Check sheet for the modelled part. Datum: model origin and axes. Units: mm. A direction names the side the tool comes from. Give positions to 0.01 mm unless a question says otherwise; leave off trailing zeros. Order: outer loops, then holes, each group sorted by start corner. A loop starts at its lowest first (then second) coordinate and runs counter-clockwise, first axis right, second up. Notation, with made-up numbers: (-32.5, 19.5) -> (0.5, 19.5) arc R10 ccw to (0.5, 34.5) -> close; hole circle Ø10 at (62, 13.25). An arc over 180 degrees is marked (long way). One line per question, with ' | ' between items.
```python
from build123d import *

# Parameters (mm, degrees)
EXTRUDE_1_DEPTH              = 7
CUT_EXTRUDE_1_DEPTH          = 4
HOLE_WIZARD_M3_1_D           = 3.4
HOLE_WIZARD_M3_1_DEPTH       = 7.5
HOLE_WIZARD_M3_1_CSINK_D     = 6.72
HOLE_WIZARD_M3_1_CSINK_ANGLE = 90
HOLE_WIZARD_M3_1_TIP         = 1.021463052
HOLE_WIZARD_1_D              = 4.15
CUT_EXTRUDE_2_DEPTH          = 4
CHAMFER_1_SIZE               = 0.5


with BuildPart() as part:
    # 草图1 → 凸台-拉伸1 (new body)
    with BuildSketch(Plane(origin=(0, 0, 0), x_dir=(1, 0, 0), z_dir=(0, 1, 0))):
        with BuildLine():
            Line((0, 5), (9, 5))
            ThreePointArc((9, 5), (14, 0), (9, -5))
            Line((9, -5), (0, -5))
            ThreePointArc((0, -5), (-5, 0), (0, 5))
        make_face()
    extrude(amount=EXTRUDE_1_DEPTH)

    # 草图2 → 切除-拉伸1 (cut)
    with BuildSketch(Plane(origin=(0, 7, 0), x_dir=(1, 0, 0), z_dir=(0, 1, 0))):
        with BuildLine():
            ThreePointArc((-1.5, 2), (-2.5, 0), (-1.5, -2))
            Line((-1.5, -2), (1.5, -2))
            ThreePointArc((1.5, -2), (2.236067977, -1.118033989), (2.5, 0))
            ThreePointArc((2.5, 0), (2.236067977, 1.118033989), (1.5, 2))
            Line((1.5, 2), (-1.5, 2))
        make_face()
    extrude(amount=-CUT_EXTRUDE_1_DEPTH, mode=Mode.SUBTRACT)

    # M3 六角凹锥坑螺钉的锥形沉头孔1
    with Locations(Plane(origin=(0, 0, 0), x_dir=(-1, 0, 0), z_dir=(0, -1, 0))):
        with Locations((0, 0)):
            CounterSinkHole(HOLE_WIZARD_M3_1_D / 2, HOLE_WIZARD_M3_1_CSINK_D / 2, depth=HOLE_WIZARD_M3_1_DEPTH, counter_sink_angle=HOLE_WIZARD_M3_1_CSINK_ANGLE)
            with Locations((0, 0, -(HOLE_WIZARD_M3_1_DEPTH + HOLE_WIZARD_M3_1_TIP / 2))):  # 118° drill point
                Cone(0, HOLE_WIZARD_M3_1_D / 2, HOLE_WIZARD_M3_1_TIP, mode=Mode.SUBTRACT)

    # 孔1 (through all)
    with Locations(Plane(origin=(0, 0, 0), x_dir=(-1, 0, 0), z_dir=(0, -1, 0))):
        with Locations((-9, 0)):
            Hole(HOLE_WIZARD_1_D / 2)

    # 草图7 → 切除-拉伸2 (cut)
    with BuildSketch(Plane(origin=(0, 7, 0), x_dir=(1, 0, 0), z_dir=(0, 1, 0))):
        Polygon((12.348631561, 0), (10.674315781, 2.9), (7.325684219, 2.9), (5.651368439, 0), (7.325684219, -2.9), (10.674315781, -2.9), align=None)
    extrude(amount=-CUT_EXTRUDE_2_DEPTH, mode=Mode.SUBTRACT)

    # 倒角1
    chamfer_1_edges = [part.edges().sort_by_distance(p)[0] for p in [
        (14, 7, 0),
        (4.5, 7, -5),
        (-5, 7, 0),
        (4.5, 0, -5),
        (14, 0, 0),
        (4.5, 0, 5),
        (-5, 0, 0),
        (4.5, 7, 5),
    ]]
    chamfer(chamfer_1_edges, length=CHAMFER_1_SIZE)


solid = part.part
```
Q1. Mould release check, pull along X, two halves, no side actions. Record for faces 3 (the face through (6.5, 5.03, -1.47)), 4 (the face through (14, 3, 0)), 5 (the face through (5, 3, 5)): pulls with the +X half, pulls with the -X half, needs draft (parallel to the pull), parting line crosses it, or undercut.
Result sheet:
face 3: undercut | face 4: pulls with the +X half | face 5: needs draft
Q2. Access from +Z, -Z, +X, -X, +Y, -Y to the whole of each face (thin tool, end or side, straight path). Record for faces 1 (the face through (0, 5, -2)), 2 (the face through (-5, 3, 0)).
Result sheet:
face 1: +Y | face 2: -X, +Y, -Y
Q3. Depth check by flat-ended pin: pin 1 Ø3 at (x, y) = (-3, 3.5) entering from -Z. Enter the tip coordinate at first touch or a pass-through.
Result sheet:
pin 1: stops at z = -4.77
Q4. Thickness scan on line 1 (X direction, y = 4, z = -1); line 2 (X direction, y = 1.75, z = 0.5); line 3 (Z direction, x = 7.5, y = 5.5). Record the ranges inside material, lowest first.
Result sheet:
line 1: x = -4.9 to -2.29, 2.29 to 6.23, 11.77 to 13.9 | line 2: x = -4.97 to -1.62, 1.62 to 6.99, 11.01 to 13.97 | line 3: z = -5 to -2.9, 2.9 to 5
Q5. Section check A-A (y = 5.5). Enter the section's corners in (x, z).
Result sheet:
outline: (0, -5) -> (9, -5) arc R5 ccw to (9, 5) -> (0, 5) arc R5 ccw to start; hole (-1.5, -2) -> (1.5, -2) arc R2.5 ccw to (1.5, 2) -> (-1.5, 2) arc R2.5 ccw to start; hole (5.65, 0) -> (7.33, -2.9) -> (10.67, -2.9) -> (12.35, 0) -> (10.67, 2.9) -> (7.33, 2.9) -> close
Q6. Section check C-C (z = 0.75). Count the separate pieces of the cut face and the enclosed holes in it, and give its area (3 significant figures).
Result sheet:
separate pieces: 3 | enclosed holes: 0 | area: 65.6 mm2
Q7. Section check B-B (x = 8). Enter the section's corners in (y, z).
Result sheet:
outline: (0, -4.5) -> (0.5, -5) -> (6.5, -5) -> (7, -4.5) -> (7, -2.9) -> (3, -2.9) -> (3, -1.82) -> (0, -1.82) -> close; (0, 1.82) -> (3, 1.82) -> (3, 2.9) -> (7, 2.9) -> (7, 4.5) -> (6.5, 5) -> (0.5, 5) -> (0, 4.5) -> close
Q8. Section check D-D (y = 1). Enter the section's corners in (x, z) (3 decimals), and give its area (3 significant figures).
Result sheet:
outline: (0, -5) -> (9, -5) arc R5 ccw to (9, 5) -> (0, 5) arc R5 ccw to start; hole circle Ø4.72 at (0, 0); hole circle Ø4.15 at (9, 0) | area: 138 mm2
